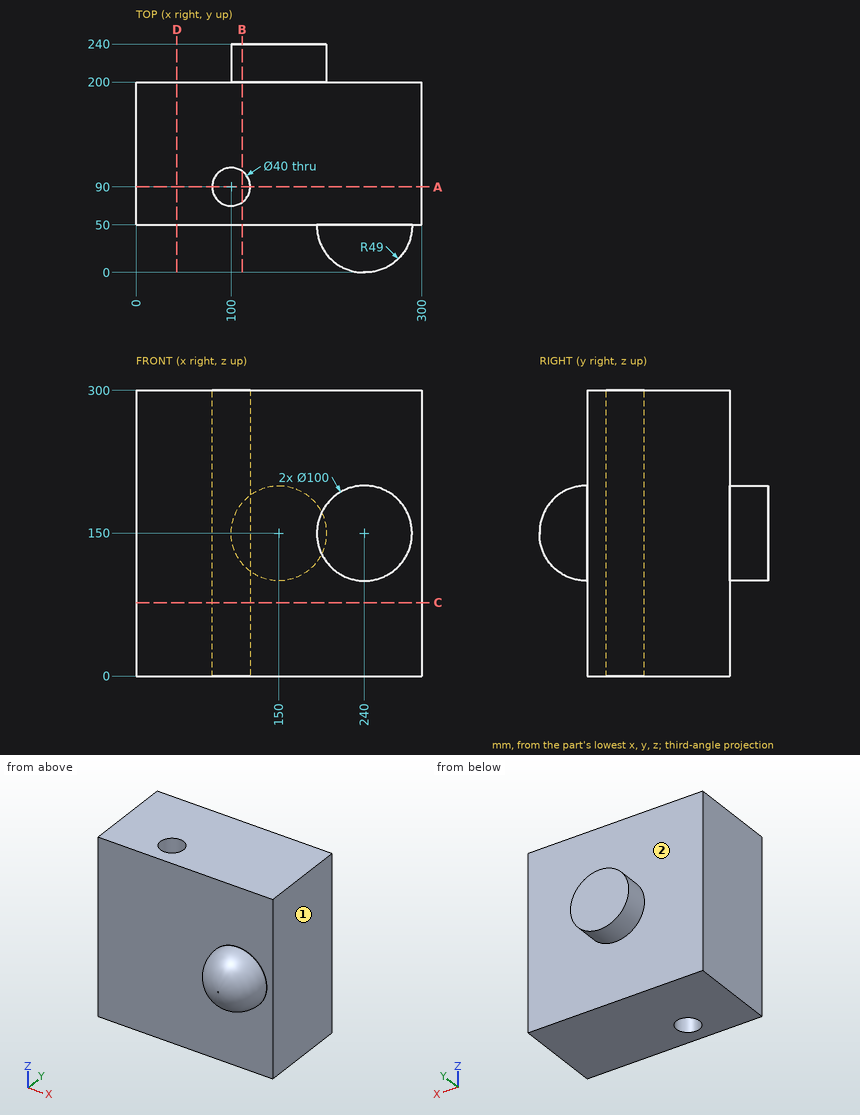
The figure shows three views and two pictorial views of one solid part (mm, origin at its lowest corner). Answer the questions. A direction names the side the tool comes from. Give positions to 0.01 mm unless a question says otherwise; leave off trailing zeros. Write each loop counter-clockwise with the first axis right and the second up, starting at its lowest first coordinate (ties: lowest second). Pieces come first, ordered by that corner, then holes. Notation, with made-up numbers: (-40, 61.5) -> (-19, 61.5) arc R16 cw to (-19, 65.5) -> close; hole circle Ø10 at (84, 15.5). An arc over 180 degrees is marked (long way). Use one line per item in the form item = value.
1) A tool of negligible diameter and unlimited length cuts with its end or side. For the marked faces 1 and 2, from which of +Z, -Z, +X, -X, +Y, -Y can it reach the whole face along a straight path? Write none if from no direction.
Result:
face_1 = +Z, -Z, +X, +Y, -Y
face_2 = +Y
2) Straight lines are drawn through the part: probe 1 along Y at (x, z) = (100, 130); probe 2 along Y at (x, z) = (238.5, 207.5); probe 3 along Y at (x, z) = (155.5, 187). For each, find the intervals that lie inside material, in ascending order.
Result:
probe_1 = 50 to 70, 110 to 200
probe_2 = 50 to 200
probe_3 = 50 to 240
3) Each of these flat-tipped pins is pushed along its axis until it touches: P1, Ø2, axis at x = 228, z = 246, coming from the +Y side; P2, Ø5, axis at y = 160, z = 183.5, coming from the -X side; P3, Ø2, axis at x = 175.5, z = 182.5, coming from the -Y side. Where does it stop, or does it pass through?
Result:
P1 = 200
P2 = 0
P3 = 50
4) Section C-C on z = 77 is taken. Write down the section's boundary in (x, y), plus the area to 3 significant figures.
Result:
outline = (0, 50) -> (300, 50) -> (300, 200) -> (0, 200) -> close; hole circle Ø40 at (100, 90)
area = 43,700 mm²
5) Section D-D on x = 43 is taken. Write down the section's boundary in (y, z), plus the area to 3 significant figures.
Result:
outline = (50, 0) -> (200, 0) -> (200, 300) -> (50, 300) -> close
area = 45,000 mm²
6) Section A-A on y = 90 is taken. Write down the section's boundary in (x, z).
Result:
outline = (0, 0) -> (80, 0) -> (80, 300) -> (0, 300) -> close; (120, 0) -> (300, 0) -> (300, 300) -> (120, 300) -> close
7) Section B-B on x = 111.5 is taken. Write down the section's boundary in (y, z), plus the area to 3 significant figures.
Result:
outline = (50, 0) -> (73.64, 0) -> (73.64, 300) -> (50, 300) -> close; (106.36, 0) -> (200, 0) -> (200, 118.1) -> (240, 118.1) -> (240, 181.9) -> (200, 181.9) -> (200, 300) -> (106.36, 300) -> close
area = 37,700 mm²
